Work out the finished part from the listing and answer in its coordinate system (mm). Face numbers are marked on the shaded views. Round coordinates to 2 decimals unless told otherwise and drop trailing zeros. Write each loop counter-clockwise with the first axis right and the second up, starting at its lowest first coordinate (ties: lowest second). Pieces come first, ordered by that corner, then holes.
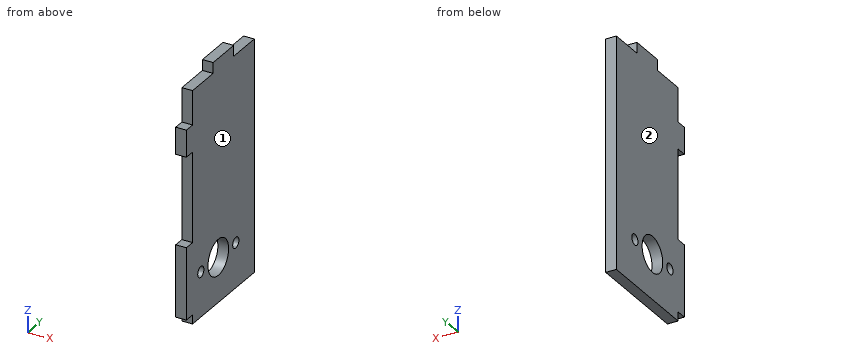
Autodesk Inventor part; units mm, degrees
ref_plane "YZ Plane" through (0, 0, 0) normal (1, 0, 0) x (0, 1, 0)
ref_plane "XZ Plane" through (0, 0, 0) normal (0, 1, 0) x (-1, 0, 0)
ref_plane "XY Plane" through (0, 0, 0) normal (0, 0, 1) x (1, 0, 0)
sketch "Sketch1" plane through (0, 0, 0) normal (1, 0, 0) x (0, 1, 0)
  line L0 (15, 52) -> (-15, 52)
  line L1 (-15, 52) -> (-15, -12.5)
  line L2 (-15, -12.5) -> (15, -12.5)
  line L3 (15, -12.5) -> (15, 52)
  line L4 (-15, 10) -> (-18, 10)
  line L5 (-18, 10) -> (-18, -10)
  line L6 (-18, -10) -> (-15, -10)
  line L7 (-15, -10) -> (-15, 10)
  line L8 (-15, 42.5) -> (-18, 42.5)
  line L9 (-18, 42.5) -> (-18, 35)
  line L10 (-18, 35) -> (-15, 35)
  line L11 (-15, 35) -> (-15, 42.5)
  point P0 (0, 0)
  point P1 (0, -12.5)
  point P2 (-18, 0)
  dimension "d0" = 52
  dimension "d1" = 12.5
  dimension "d2" = 3
  dimension "d3" = 20
  dimension "d4" = 7.5
  dimension "d5" = 25
  dimension "d8" = 30
extrude "Extrusion1" add sketch "Sketch1" along normal blind 3
sketch "Sketch2" plane through (3, 0, 0) normal (1, 0, 0) x (0, 0, -1)
  circle A0 centre (0, -2.5) radius 5
  circle A1 centre (0, 6) radius 1.5
  circle A2 centre (0, -11) radius 1.5
  line L0 (-10, -18) -> (10, -18)
  line L1 (-35, -15) -> (-10, -15)
  point P0 (0, -18)
  dimension "d9" = 10
  dimension "d10" = 3
  dimension "d11" = 3
  dimension "d12" = 17
  dimension "d13" = 8.5
  dimension "d20" = 12.5
extrude "Extrusion2" cut sketch "Sketch2" against normal blind 3
sketch "Sketch3" plane through (3, 0, 0) normal (1, 0, 0) x (0, 0, -1)
  line L0 (-52, 15) -> (-52, -15)
  line L1 (-52, 5) -> (-55, 5)
  line L2 (-55, 5) -> (-55, -5)
  line L3 (-55, -5) -> (-52, -5)
  line L4 (-52, -5) -> (-52, 5)
  point P0 (0, 0)
  point P1 (-55, 0)
  dimension "d16" = 3
  dimension "d17" = 10
extrude "Extrusion3" add sketch "Sketch3" against normal blind 3
properties part number "Motor support"
Q1. Given pin 1 (9 mm diameter, centred on y = -2.5, z = 0, fed in from +X); pin 2 (0.9 mm diameter, centred on x = 1, z = 48, fed in from -Y); pin 3 (1.5 mm diameter, centred on x = 1, y = -16, fed in from +Z), each flat-ended and moving along its own axis, determine where each tip first touches the part or whether it passes through.
Q2. Find section B-B (y = -2.5). Determine the outline of the cut face in (x, z), plus the area to 4 significant figures.
Q3. Find section C-C (x = 1.6). Determine the outline of the cut face in (y, z), plus the area to 3 significant figures.
Q4. Find the intervals of material crossed by L1, parallel to Y at x = 2.2, z = 0; L2, parallel to Y at x = 0.8, z = 48; L3, parallel to Z at x = 1.2, y = 10.5, in increasing order.
Q5. Find section A-A (z = 0). Determine the outline of the cut face in (x, y), plus the area to 3 significant figures.
Q6. The mould has two halves that part along X. Classify the marked faces 1 and 2: +X half, -X half, draft (parallel to the pull), parting line (faces both ways), or undercut.
Q7. Find section D-D (y = -11). Determine the outline of the cut face in (x, z), plus the area to 4 significant figures.
Report:
1. pin 1: passes through
1. pin 2: stops at y = -15
1. pin 3: stops at z = 42.5
2. outline: (0, -12.5) - (3, -12.5) - (3, -5) - (0, -5) - close; (0, 5) - (3, 5) - (3, 55) - (0, 55) - close
2. area: 172.5 mm2
3. outline: (-18, -10) - (-15, -10) - (-15, -12.5) - (15, -12.5) - (15, 52) - (5, 52) - (5, 55) - (-5, 55) - (-5, 52) - (-15, 52) - (-15, 42.5) - (-18, 42.5) - (-18, 35) - (-15, 35) - (-15, 10) - (-18, 10) - close; hole circle Ø3 at (-11, 0); hole circle Ø10 at (-2.5, 0); hole circle Ø3 at (6, 0)
3. area: 1,950 mm2
4. L1: y = -18 to -12.5, -9.5 to -7.5, 2.5 to 4.5, 7.5 to 15
4. L2: y = -15 to 15
4. L3: z = -12.5 to 52
5. outline: (0, -18) - (3, -18) - (3, -12.5) - (0, -12.5) - close; (0, -9.5) - (3, -9.5) - (3, -7.5) - (0, -7.5) - close; (0, 2.5) - (3, 2.5) - (3, 4.5) - (0, 4.5) - close; (0, 7.5) - (3, 7.5) - (3, 15) - (0, 15) - close
5. area: 51.0 mm2
6. face 1: +X half
6. face 2: -X half
7. outline: (0, -12.5) - (3, -12.5) - (3, -1.5) - (0, -1.5) - close; (0, 1.5) - (3, 1.5) - (3, 52) - (0, 52) - close
7. area: 184.5 mm2
